Verification items for the finished model (mm, model axes). Round coordinates to 2 decimals unless told otherwise and drop trailing zeros. Write each loop counter-clockwise with the first axis right and the second up, starting at its lowest first coordinate (ties: lowest second). Pieces come first, ordered by that corner, then holes. Notation, with made-up numbers: M 16,43.25 L 42,43.25 A21 ccw 42,55.25 Z; hole C -33,75.25 d6. An arc over 180 degrees is marked long. One line per item, written item: value. Start each with the question number.
Item 1: Gauge pin test, flat end, axial feed: pin 1 (2.5 mm diameter, centred on x = 30.5, y = -42.7, fed in from -Z). Record the tip position at first contact, or that the pin passes through.
Item 2: Section check B-B, the plane x = 30.5. Record the cut outline in (y, z), then the cut area to 3 significant figures.
Item 3: Thickness scan on probe 1 along Y at (x, z) = (-30.5, 0.4). Record the ranges inside material, lowest first. Write a range as from..to.
Item 4: Section check A-A, the plane y = -42.7. Record the cut outline in (x, z).
Item 5: Draft check along Y on faces 1 (the face through (-1, 1, 0)), 2 (the face through (-30.175, 42.536, 0.493)). Enter one of: +Y half, -Y half, draft (parallel to the pull), parting line (faces both ways), or undercut.
from build123d import *

# Parameters (mm, degrees)
SKETCH1_W                    = 93.4
SKETCH1_H                    = 93.4
BOSS_EXTRUDE1_DEPTH          = 1
F_3_0_3_DIAMETER_HOLE1_D     = 3
F_3_0_3_DIAMETER_HOLE1_DEPTH = 1


with BuildPart() as part:
    # Sketch1 → Boss-Extrude1 (new body)
    with BuildSketch(Plane.XY):
        Rectangle(SKETCH1_W, SKETCH1_H)
    extrude(amount=BOSS_EXTRUDE1_DEPTH)

    # Ø3.0 (3) Diameter Hole1
    with Locations(Plane.XY.offset(1)):
        with Locations((-30.5, -47.3), (30.5, -47.3), (30.5, -42.7), (-30.5, -42.7), (-30.5, 44), (30.5, 44), (-30.5, -66), (30.5, -66)):
            Hole(F_3_0_3_DIAMETER_HOLE1_D / 2, depth=F_3_0_3_DIAMETER_HOLE1_DEPTH)


solid = part.part
Response values:
1. pin 1: passes through
2. outline: M -45.8,0 L -44.2,0 L -44.2,1 L -45.8,1 Z; M -41.2,0 L 42.5,0 L 42.5,1 L -41.2,1 Z; M 45.5,0 L 46.7,0 L 46.7,1 L 45.5,1 Z
2. area: 86.5 mm2
3. probe 1: y = -45.8..-44.2, -41.2..42.5, 45.5..46.7
4. outline: M -46.7,0 L -32,0 L -32,1 L -46.7,1 Z; M -29,0 L 29,0 L 29,1 L -29,1 Z; M 32,0 L 46.7,0 L 46.7,1 L 32,1 Z
5. face 1: draft
5. face 2: undercut
